Verification items for the finished model (mm, model axes). Face numbers are marked on the shaded views. A direction names the side the tool comes from. Coordinates: 2 decimals unless noted, no trailing zeros. Order: outer loops, then holes, each group sorted by start corner. A loop starts at its lowest first (then second) coordinate and runs counter-clockwise, first axis right, second up. Notation, with made-up numbers: M 19,2 L 55,2 A14 cw 55,10 Z; hole C 53.25,70 d8. An arc over 180 degrees is marked long. Answer as a JSON object with one key per item and string values. Group by question number.
(1) Mould release check, pull along Z, two halves, no side actions. Record for the marked faces 1, 2, 3 and 4: released by +Z, released by -Z, zero draft, split by the parting line, or undercut.
(2) Cross-section at C-C (z = 2.75). Enter the section's corners in (x, y) (3 decimals), plus the area to 3 significant figures.
(3) Access from +Z, -Z, +X, -X, +Y, -Y to the whole of each face (thin tool, end or side, straight path). Record for the marked faces 5 and 6.
(4) Cross-section at B-B (y = -2). Enter the section's corners in (x, z) (3 decimals).
(5) Material ranges on line 1 (X direction, y = -12.25, z = 8.5); line 2 (Z direction, x = 5.75, y = -2) (3 decimals); line 3 (Y direction, x = 2.5, z = 1.65) (3 decimals), recorded low to high.
(6) Cross-section at D-D (z = 9.5). Enter the section's corners in (x, y) (3 decimals).
(7) Cross-section at A-A (x = 2.5). Enter the section's corners in (y, z) (3 decimals).
(8) Gauge pin test, flat ends, axial feed: pin 1 Ø3 at (x, z) = (16.52, 8.56) entering from +Y; pin 2 Ø4 at (x, z) = (15, 8) entering from +Y. Record the tip position at first contact, or that the pin passes through.
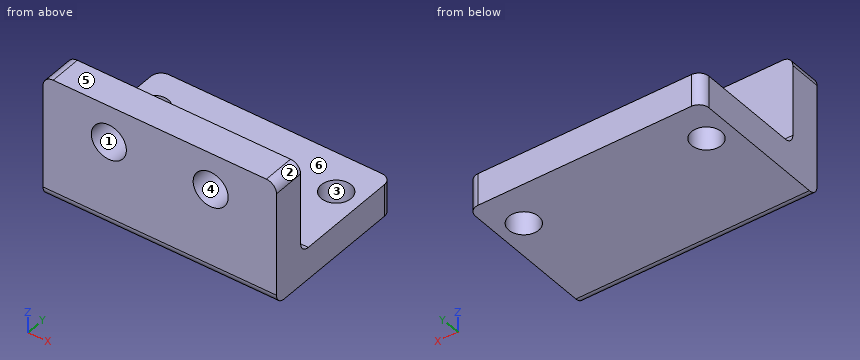
from build123d import *

# Parameters (mm, degrees)
SKETCH1_W             = 23
SKETCH1_H             = 10
SKETCH1_R             = 1.4732
SKETCH1_H_2           = 3.175
SKETCH1_H_3           = 2
BOSS_EXTRUDE1_DEPTH   = 3.175
BOSS_EXTRUDE2_START   = 3.175
SKETCH1_3_W           = 23
SKETCH1_3_H           = 3.175
BOSS_EXTRUDE2_DEPTH   = 9
F_8_32_TAPPED_HOLE1_D = 3.4544
FILLET1_R             = 1


with BuildPart() as part:
    # Sketch1 → Boss-Extrude1 (new body)
    # profile 1 of 3: a face of its own
    with BuildSketch(Plane.XY):
        with Locations((11.5, -5)):
            Rectangle(SKETCH1_W, SKETCH1_H)
        with Locations((2.5, -2)):
            Circle(SKETCH1_R, mode=Mode.SUBTRACT)
        with Locations((20.5, -2)):
            Circle(SKETCH1_R, mode=Mode.SUBTRACT)
    # profile 2 of 3: a face of its own
    with BuildSketch(Plane.XY):
        with Locations((11.5, -11.5875)):
            Rectangle(SKETCH1_W, SKETCH1_H_2)
    # profile 3 of 3: a face of its own
    with BuildSketch(Plane.XY):
        with Locations((11.5, 1)):
            Rectangle(SKETCH1_W, SKETCH1_H_3)
    extrude(amount=BOSS_EXTRUDE1_DEPTH)

    # Sketch1<3> → Boss-Extrude2 (add)
    with BuildSketch(Plane.XY.offset(BOSS_EXTRUDE2_START)):
        with Locations((11.5, -11.5875)):
            Rectangle(SKETCH1_3_W, SKETCH1_3_H)
    extrude(amount=BOSS_EXTRUDE2_DEPTH)

    # #8-32 Tapped Hole1 (through all)
    with Locations(Plane(origin=(6.4835, -10, 8.5555), x_dir=(1, 0, 0), z_dir=(0, 1, 0))):
        with Locations((0, 0), (10.033, 0)):
            Hole(F_8_32_TAPPED_HOLE1_D / 2)

    # Fillet1
    fillet1_edges = [part.edges().sort_by_distance(p)[0] for p in [
        (0, 2, 1.5875),
        (23, 2, 1.5875),
        (0, -11.5875, 12.175),
        (11.5, -10, 3.175),
        (23, -11.5875, 12.175),
        (11.5, -13.175, 0),
    ]]
    fillet(fillet1_edges, radius=FILLET1_R)


solid = part.part
Taken from the geometry:
{
 "1": {"face 1": "undercut", "face 2": "released by +Z", "face 3": "zero draft", "face 4": "undercut"},
 "2": {"outline": "M 0,-13.175 L 23,-13.175 L 23,1 A1 ccw 22,2 L 1,2 A1 ccw 0,1 Z; hole C 2.5,-2 d2.946; hole C 20.5,-2 d2.946", "area": "335 mm²"},
 "3": {"face 5": "+Z, +X, -X, +Y, -Y", "face 6": "+Z, +X, -X, +Y"},
 "4": {"outline": "M 0,0 L 1.027,0 L 1.027,3.175 L 0,3.175 Z; M 3.973,0 L 19.027,0 L 19.027,3.175 L 3.973,3.175 Z; M 21.973,0 L 23,0 L 23,3.175 L 21.973,3.175 Z"},
 "5": {"line 1": "x = 0 to 4.76, 8.21 to 14.79, 18.24 to 23", "line 2": "z = 0 to 3.175", "line 3": "y = -13.175 to -3.473, -0.527 to 2"},
 "6": {"outline": "M 0,-13.175 L 5.037,-13.175 L 5.037,-10 L 0,-10 Z; M 7.93,-13.175 L 15.07,-13.175 L 15.07,-10 L 7.93,-10 Z; M 17.963,-13.175 L 23,-13.175 L 23,-10 L 17.963,-10 Z"},
 "7": {"outline": "M -13.175,1 A1 ccw -12.175,0 L -3.473,0 L -3.473,3.175 L -9,3.175 A1 cw -10,4.175 L -10,12.175 L -13.175,12.175 Z; M -0.527,0 L 2,0 L 2,3.175 L -0.527,3.175 Z"},
 "8": {"pin 1": "passes through", "pin 2": "stops at y = -10"}
}
